Can you work these out from the model? Positions are in its coordinate system, mm. A direction names the side the tool comes from. Coordinates: 2 decimals unless noted, no trailing zeros. Order: outer loops, then holes, each group sorted by start corner. A loop starts at its lowest first (then second) coordinate and runs counter-clockwise, first axis right, second up. Notation, with made-up numbers: (73, 38) -> (105, 38) arc R24 ccw to (105, 71) -> close; hole circle Ø3 at (15, 69.5). An arc over 180 degrees is marked (long way). Write item = value, one per line. Start each with the question number.
from build123d import *

# Parameters (mm, degrees)
SKETCH1_W                       = 76.2
SKETCH1_H                       = 50.8
SKETCH1_W_2                     = 69.85
SKETCH1_H_2                     = 44.45
BOSS_EXTRUDE1_DEPTH             = 101.6
F_7_0_201_DIAMETER_HOLE1_REACH  = 121.812
F_7_0_201_DIAMETER_HOLE1_BORE_R = 2.5527
F_1_4_0_25_DIAMETER_HOLE1_D     = 6.35
F_1_4_0_25_DIAMETER_HOLE1_DEPTH = 3.175
CUT_EXTRUDE1_REACH              = 121.812
SKETCH8_R                       = 12.7


with BuildPart() as part:
    # Sketch1 → Boss-Extrude1 (new body)
    with BuildSketch(Plane.XY):
        Rectangle(SKETCH1_W, SKETCH1_H)
        Rectangle(SKETCH1_W_2, SKETCH1_H_2, mode=Mode.SUBTRACT)
    extrude(amount=BOSS_EXTRUDE1_DEPTH)

    # #7 (0.201) Diameter Hole1 bore → #7 (0.201) Diameter Hole1 (cut, up to next)
    with BuildSketch(Plane(origin=(0, 25.4, 0), x_dir=(1, 0, 0), z_dir=(0, 1, 0)), mode=Mode.PRIVATE) as f_7_0_201_diameter_hole1_sk1:
        with Locations((-27.0002, -50.8)):
            Circle(F_7_0_201_DIAMETER_HOLE1_BORE_R)
    f_7_0_201_diameter_hole1_tool1 = extrude(f_7_0_201_diameter_hole1_sk1.sketch, amount=-F_7_0_201_DIAMETER_HOLE1_REACH, mode=Mode.PRIVATE) & part.part
    # #7 (0.201) Diameter Hole1 bore → #7 (0.201) Diameter Hole1 (cut, up to next)
    with BuildSketch(Plane(origin=(0, 25.4, 0), x_dir=(1, 0, 0), z_dir=(0, 1, 0)), mode=Mode.PRIVATE) as f_7_0_201_diameter_hole1_sk2:
        with Locations((0, -23.7998)):
            Circle(F_7_0_201_DIAMETER_HOLE1_BORE_R)
    f_7_0_201_diameter_hole1_tool2 = extrude(f_7_0_201_diameter_hole1_sk2.sketch, amount=-F_7_0_201_DIAMETER_HOLE1_REACH, mode=Mode.PRIVATE) & part.part
    # #7 (0.201) Diameter Hole1 bore → #7 (0.201) Diameter Hole1 (cut, up to next)
    with BuildSketch(Plane(origin=(0, 25.4, 0), x_dir=(1, 0, 0), z_dir=(0, 1, 0)), mode=Mode.PRIVATE) as f_7_0_201_diameter_hole1_sk3:
        with Locations((27.0002, -50.8)):
            Circle(F_7_0_201_DIAMETER_HOLE1_BORE_R)
    f_7_0_201_diameter_hole1_tool3 = extrude(f_7_0_201_diameter_hole1_sk3.sketch, amount=-F_7_0_201_DIAMETER_HOLE1_REACH, mode=Mode.PRIVATE) & part.part
    # #7 (0.201) Diameter Hole1 bore → #7 (0.201) Diameter Hole1 (cut, up to next)
    with BuildSketch(Plane(origin=(0, 25.4, 0), x_dir=(1, 0, 0), z_dir=(0, 1, 0)), mode=Mode.PRIVATE) as f_7_0_201_diameter_hole1_sk4:
        with Locations((0, -77.8002)):
            Circle(F_7_0_201_DIAMETER_HOLE1_BORE_R)
    f_7_0_201_diameter_hole1_tool4 = extrude(f_7_0_201_diameter_hole1_sk4.sketch, amount=-F_7_0_201_DIAMETER_HOLE1_REACH, mode=Mode.PRIVATE) & part.part
    add(f_7_0_201_diameter_hole1_tool1.solids().sort_by_distance((-27.0002, 25.4, 50.8))[0], mode=Mode.SUBTRACT)
    add(f_7_0_201_diameter_hole1_tool2.solids().sort_by_distance((0, 25.4, 23.7998))[0], mode=Mode.SUBTRACT)
    add(f_7_0_201_diameter_hole1_tool3.solids().sort_by_distance((27.0002, 25.4, 50.8))[0], mode=Mode.SUBTRACT)
    add(f_7_0_201_diameter_hole1_tool4.solids().sort_by_distance((0, 25.4, 77.8002))[0], mode=Mode.SUBTRACT)

    # 1/4 (0.25) Diameter Hole1
    with Locations(Plane(origin=(0, -25.4, 0), x_dir=(-1, 0, 0), z_dir=(0, -1, 0))):
        with Locations((25.4, -25.4), (25.4, -76.2), (-25.4, -76.2), (-25.4, -25.4)):
            Hole(F_1_4_0_25_DIAMETER_HOLE1_D / 2, depth=F_1_4_0_25_DIAMETER_HOLE1_DEPTH)

    # Sketch8 → Cut-Extrude1 (cut, up to next)
    with BuildSketch(Plane(origin=(0, 25.4, 0), x_dir=(1, 0, 0), z_dir=(0, 1, 0)), mode=Mode.PRIVATE) as cut_extrude1_sk1:
        with Locations(Location((0, -50.8, 0), (0, 0, 270))):
            Circle(SKETCH8_R)
    cut_extrude1_tool1 = extrude(cut_extrude1_sk1.sketch, amount=-CUT_EXTRUDE1_REACH, mode=Mode.PRIVATE) & part.part
    add(cut_extrude1_tool1.solids().sort_by_distance((0, 25.4, 50.8))[0], mode=Mode.SUBTRACT)


solid = part.part
(1) Imagine slicing it at A-A (z = 81.5). Write out the boundary of the cut face in (x, y) (3 decimals).
(2) Thinking about a two-plate mould opening in Z: for faces 1 (the face through (-0.33, 23.83, 21.27)), 2 (the face through (-7.7, 23.8, 40.7)), 3 (the face through (-1, -25.4, 50)), 4 (the face through (-3, -22.5, 101.6)), which applies, +Z half, -Z half, draft (parallel to the pull), parting line (faces both ways), or undercut?
(3) For faces 5 (the face through (24.97, 23.83, 52.35)), 6 (the face through (34.925, 0, 50)), 7 (the face through (-38.1, 0, 50)), 8 (the face through (26.9, -23.8, 79)), which set-ups out of +Z, -Z, +X, -X, +Y, -Y let a thin tool reach every point of the face, with its end or its side?
(4) Imagine slicing it at B-B (x = -15). Write out the boundary of the cut face in (y, z) (3 decimals), plus the area to 3 significant figures.
(5) For P1, Ø3, axis at x = 0, z = 77.8, coming from the +Y side (3 decimals); P2, Ø4, axis at x = 25.4, z = 76.2, coming from the -Y side (3 decimals), each with a flat end and sliding along its axis, tell me the tip position at first contact or that it passes through.
(6) Imagine slicing it at D-D (z = 50.8). Write out the boundary of the cut face in (x, y) (1 decimal).
(7) If I drill on L1, parallel to X at y = -23.05, z = 76.2 (3 decimals); L2, parallel to Z at x = 25, y = -23; L3, parallel to Y at x = 10.5, z = 5 (3 decimals), over which ranges is the centre line in solid material (lowest first)? Write a range as from..to.
(8) Imagine slicing it at C-C (y = 7). Write out the boundary of the cut face in (x, z) (3 decimals), plus the area to 3 significant figures.
Result set:
q1.outline = (-38.1, -25.4) -> (38.1, -25.4) -> (38.1, 25.4) -> (-38.1, 25.4) -> close; hole (-34.925, -22.225) -> (34.925, -22.225) -> (34.925, 22.225) -> (-34.925, 22.225) -> close
q2.face_1 = undercut
q2.face_2 = undercut
q2.face_3 = draft
q2.face_4 = +Z half
q3.face_5 = +Y
q3.face_6 = +Z, -Z
q3.face_7 = +Z, -Z, -X, +Y, -Y
q3.face_8 = -Y
q4.outline = (-25.4, 0) -> (-22.225, 0) -> (-22.225, 101.6) -> (-25.4, 101.6) -> close; (22.225, 0) -> (25.4, 0) -> (25.4, 101.6) -> (22.225, 101.6) -> close
q4.area = 645 mm2
q5.P1 = -22.225
q5.P2 = 22.225
q6.outline = (-38.1, -25.4) -> (38.1, -25.4) -> (38.1, 25.4) -> (29.6, 25.4) -> (29.6, 22.2) -> (34.9, 22.2) -> (34.9, -22.2) -> (-34.9, -22.2) -> (-34.9, 22.2) -> (-29.6, 22.2) -> (-29.6, 25.4) -> (-38.1, 25.4) -> close; (-24.4, 22.2) -> (-12.7, 22.2) -> (-12.7, 25.4) -> (-24.4, 25.4) -> close; (12.7, 22.2) -> (24.4, 22.2) -> (24.4, 25.4) -> (12.7, 25.4) -> close
q7.L1 = -38.1..-28.575, -22.225..22.225, 28.575..38.1
q7.L2 = 0..22.25, 28.55..73.05, 79.35..101.6
q7.L3 = -25.4..-22.225, 22.225..25.4
q8.outline = (-38.1, 0) -> (-34.925, 0) -> (-34.925, 101.6) -> (-38.1, 101.6) -> close; (34.925, 0) -> (38.1, 0) -> (38.1, 101.6) -> (34.925, 101.6) -> close
q8.area = 645 mm2
